from build123d import *

# Parameters (mm, degrees)
BOSS_EXTRUDE5_DEPTH  = 430
SKETCH6_W            = 220
SKETCH6_H            = 410
CUT_EXTRUDE5_DEPTH   = 430
SKETCH7_W            = 7
SKETCH7_H            = 30
BOSS_EXTRUDE6_DEPTH  = 30
SKETCH8_W            = 7
SKETCH8_H            = 30
BOSS_EXTRUDE7_DEPTH  = 30
BOSS_EXTRUDE8_DEPTH  = 28
CUT_EXTRUDE6_DEPTH   = 430
BOSS_EXTRUDE9_DEPTH  = 38.4
SKETCH12_W           = 430
SKETCH12_H           = 6
CUT_EXTRUDE7_DEPTH   = 500
SKETCH13_W           = 15.031983572
SKETCH13_H           = 10
BOSS_EXTRUDE10_DEPTH = 15
SKETCH14_W           = 14.940905272
SKETCH14_H           = 10
SKETCH14_W_2         = 5
SKETCH14_H_2         = 410
BOSS_EXTRUDE11_DEPTH = 15


with BuildPart() as part:
    # Sketch1 → Boss-Extrude5 (new body)
    with BuildSketch(Plane.XY):
        Polygon((230, 122), (0, 122), (0, 0), (50, 0), (50, 30), (28.531983572, 30), (28.531983572, 38.499978431), (20.031983572, 38.499978431), (20.031983572, 62.999978431), (47.532005141, 90.5), (182.467994859, 90.5), (182.559073159, 90.5), (210.059094728, 62.999978431), (210.059094728, 38.499978431), (209.968016428, 38.499978431), (201.559094728, 38.499978431), (201.559094728, 30), (201.468016428, 30), (180, 30), (180, 0), (230, 0), align=None)
    extrude(amount=BOSS_EXTRUDE5_DEPTH)

    # Sketch6 → Cut-Extrude5 (cut)
    with BuildSketch(Plane(origin=(0, 122, 0), x_dir=(1, 0, 0), z_dir=(0, 1, 0))):
        with Locations((115, -215)):
            Rectangle(SKETCH6_W, SKETCH6_H)
    extrude(amount=-CUT_EXTRUDE5_DEPTH, mode=Mode.SUBTRACT)

    # Sketch7 → Boss-Extrude6 (add)
    with BuildSketch(Plane.XY.offset(10)):
        with Locations((46.5, 15)):
            Rectangle(SKETCH7_W, SKETCH7_H)
        with Locations((183.5, 15)):
            Rectangle(SKETCH7_W, SKETCH7_H)
    extrude(amount=BOSS_EXTRUDE6_DEPTH)

    # Sketch8 → Boss-Extrude7 (add)
    with BuildSketch(Plane(origin=(0, 0, 420), x_dir=(-1, 0, 0), z_dir=(0, 0, -1))):
        with Locations((-183.5, 15)):
            Rectangle(SKETCH8_W, SKETCH8_H)
        with Locations((-46.5, 15)):
            Rectangle(SKETCH8_W, SKETCH8_H)
    extrude(amount=BOSS_EXTRUDE7_DEPTH)

    # Sketch9 → Boss-Extrude8 (add)
    with BuildSketch(Plane.XZ):
        Polygon((50, 430), (0, 430), (0, 0), (50, 0), (50, 40), (43, 40), (43, 10), (5, 10), (5, 420), (43, 420), (43, 390), (50, 390), align=None)
        Polygon((187, 420), (225, 420), (225, 10), (187, 10), (187, 40), (180, 40), (180, 0), (230, 0), (230, 430), (180, 430), (180, 390), (187, 390), align=None)
    extrude(amount=BOSS_EXTRUDE8_DEPTH)

    # Sketch10 → Cut-Extrude6 (cut)
    with BuildSketch(Plane(origin=(0, 0, 0), x_dir=(-1, 0, 0), z_dir=(0, 0, -1))):
        Polygon((-201.559094728, 38.499978431), (-210.059094728, 38.499978431), (-210.059094728, -28), (-180, -28), (-180, 30), (-201.559094728, 30), align=None)
        Polygon((-28.531983572, 30), (-50, 30), (-50, -28), (-20.031983572, -28), (-20.031983572, 30), (-20.031983572, 38.499978431), (-28.531983572, 38.499978431), align=None)
    extrude(amount=-CUT_EXTRUDE6_DEPTH, mode=Mode.SUBTRACT)

    # Sketch11 → Boss-Extrude9 (add)
    with BuildSketch(Plane.XZ.offset(28)):
        Polygon((230, 0), (225, 0), (210.059094728, 0), (210.059094728, 10), (225, 10), (225, 420), (210.059094728, 420), (210.059094728, 430), (230, 430), (230, 420), align=None)
        Polygon((5, 10), (5, 420), (20.031983572, 420), (20.031983572, 430), (5, 430), (0, 430), (0, 10), (0, 0), (20.031983572, 0), (20.031983572, 10), align=None)
    extrude(amount=BOSS_EXTRUDE9_DEPTH)

    # Sketch12 → Cut-Extrude7 (cut)
    with BuildSketch(Plane.ZY):
        with Locations((215, -63.4)):
            Rectangle(SKETCH12_W, SKETCH12_H)
    extrude(amount=-CUT_EXTRUDE7_DEPTH, mode=Mode.SUBTRACT)

    # Sketch13 → Boss-Extrude10 (add)
    with BuildSketch(Plane.XZ.offset(60.4)):
        with Locations((12.515991786, 425)):
            Rectangle(SKETCH13_W, SKETCH13_H)
        Polygon((5, 430), (0, 430), (0, 10), (5, 10), (5, 420), align=None)
        Polygon((5, 10), (0, 10), (0, 0), (20.031983572, 0), (20.031983572, 10), align=None)
    extrude(amount=BOSS_EXTRUDE10_DEPTH)

    # Sketch14 → Boss-Extrude11 (add)
    with BuildSketch(Plane.XZ.offset(60.4)):
        with Locations((217.529547364, 425)):
            Rectangle(SKETCH14_W, SKETCH14_H)
        with Locations((227.5, 425)):
            Rectangle(SKETCH14_W_2, SKETCH14_H)
        with Locations((227.5, 215)):
            Rectangle(SKETCH14_W_2, SKETCH14_H_2)
        Polygon((230, 0), (230, 10), (225, 10), (210.059094728, 10), (210.059094728, 0), align=None)
    extrude(amount=BOSS_EXTRUDE11_DEPTH)


solid = part.part
The listing builds one solid part. Answer for the finished solid, in the listing's coordinates (mm). A direction names the side the tool comes from. Give positions to 0.01 mm unless a question says otherwise; leave off trailing zeros. Order: outer loops, then holes, each group sorted by start corner. A loop starts at its lowest first (then second) coordinate and runs counter-clockwise, first axis right, second up. Notation, with made-up numbers: (22.25, 45.5) - (41.25, 45.5) arc R25 cw to (41.25, 61.5) - close; hole circle Ø10 at (-11.75, 10.25). An arc over 180 degrees is marked (long way). One line per item, written item: value. Start each with the question number.
1) A cutting plane is placed at C-C on y = -45. Give the vertices of the cut face in (x, z).
2) A cutting plane is placed at B-B on x = 152. Give the vertices of the cut face in (y, z), then the cut area to 3 significant figures.
3) The mould has two halves that part along Z. Classify faces 4 (the face through (5, 25, 212)), 5 (the face through (114, 90.5, 5)), 6 (the face through (107, 97, 430)), 7 (the face through (225, 25, 212)): released by +Z, released by -Z, zero draft, split by the parting line, or undercut.
4) A cutting plane is placed at A-A on z = 149. Give the vertices of the cut face in (x, y), then the cut area to 3 significant figures.
5) Given pin 1 Ø11 at (x, z) = (144, 3.5) entering from -Y, flat-ended and moving along its own axis, determine where the tip first touches the part or whether it passes through.
6) A tool of negligible diameter and unlimited length cuts with its end or side. For faces 1 (the face through (196.12, 76.94, 4.93)), 2 (the face through (116, 97, 10)), 3 (the face through (225.2, -75.4, 216)), from which of +Z, -Z, +X, -X, +Y, -Y can it reach the whole face along a straight path? Write none if from no direction.
7) Find the intervals of material crossed by L1, parallel to X at y = 112, z = 29; L2, parallel to Z at x = 142, y = 101, in increasing order.
Answer sheet:
1. outline: (0, 0) - (20.03, 0) - (20.03, 10) - (5, 10) - (5, 420) - (20.03, 420) - (20.03, 430) - (0, 430) - close; (210.06, 0) - (230, 0) - (230, 430) - (210.06, 430) - (210.06, 420) - (225, 420) - (225, 10) - (210.06, 10) - close
2. outline: (90.5, 0) - (122, 0) - (122, 10) - (90.5, 10) - close; (90.5, 420) - (122, 420) - (122, 430) - (90.5, 430) - close
2. area: 630 mm2
3. face 4: undercut
3. face 5: zero draft
3. face 6: released by +Z
3. face 7: undercut
4. outline: (0, -75.4) - (5, -75.4) - (5, 122) - (0, 122) - close; (225, -75.4) - (230, -75.4) - (230, 122) - (225, 122) - close
4. area: 1,970 mm2
5. pin 1: stops at y = 90.5
6. face 1: +Z, -Z, -Y
6. face 2: +Y, -Y
6. face 3: +Z, -Z, +X, -X, -Y
7. L1: x = 0 to 5, 225 to 230
7. L2: z = 0 to 10, 420 to 430
